Source: CAD feature listing. Evaluate the final solid. Frame: model axes, mm. Round coordinates to 2 decimals unless told otherwise and drop trailing zeros. Loops run counter-clockwise (first coordinate to the right, second up) from the corner with the lowest first, then second, coordinate; pieces in that order, holes last.
(1) Section A-A, the plane x = 55. Return the cut outline in (y, z).
(2) First-contact query: pin 1 Ø0.6 at (x, z) = (119, 13) entering from +Y. Flat tip, straight axial feed; report the tip coordinate or a pass-through.
(3) Section B-B, the plane z = 3.25. Return the cut outline in (x, y).
(4) Material intervals for probe 1 along X at (y, z) = (15.25, 2.25); probe 2 along Z at (x, y) = (36, 10.5); probe 3 along Z at (x, y) = (24.5, 0.5), sorted ascending.
```python
from build123d import *

# Parameters (mm, degrees)
SKETCH1_W           = 22
SKETCH1_H           = 18
BOSS_EXTRUDE1_DEPTH = 20
SKETCH2_W           = 12
SKETCH2_H           = 10
CUT_EXTRUDE1_DEPTH  = 13
SKETCH3_W           = 20
SKETCH3_H           = 5
BOSS_EXTRUDE2_DEPTH = 2
LPATTERN1_COUNT     = 6
LPATTERN1_PITCH     = 24
SKETCH4_W           = 20
SKETCH4_H           = 13
BOSS_EXTRUDE3_DEPTH = 2
SKETCH5_W           = 20
SKETCH5_H           = 18
BOSS_EXTRUDE4_DEPTH = 2
SKETCH6_W           = 132
SKETCH6_H           = 2
CUT_EXTRUDE2_DEPTH  = 2
SKETCH7_W           = 146
SKETCH7_H           = 20
BOSS_EXTRUDE5_DEPTH = 6


with BuildPart() as part:
    # Sketch1 → Boss-Extrude1 (new body)
    with BuildSketch(Plane.XY):
        with Locations((11, 9)):
            Rectangle(SKETCH1_W, SKETCH1_H)
    extrude(amount=BOSS_EXTRUDE1_DEPTH)

    # Sketch2 → Cut-Extrude1 (cut)
    with BuildSketch(Plane.XZ):
        with Locations((11, 10)):
            Rectangle(SKETCH2_W, SKETCH2_H)
    extrude(amount=-CUT_EXTRUDE1_DEPTH, mode=Mode.SUBTRACT)

    # Sketch3 → Boss-Extrude2 (add)
    with BuildSketch(Plane(origin=(22, 0, 0), x_dir=(0, 0, -1), z_dir=(1, 0, 0))):
        with Locations((-10, 2.5)):
            Rectangle(SKETCH3_W, SKETCH3_H)
    extrude(amount=BOSS_EXTRUDE2_DEPTH)


with BuildPart() as lpattern1_1:
    # LPattern1: pattern copy
    add(part.part.moved(Location(Vector(1, 0, 0) * (1 * LPATTERN1_PITCH))))


with BuildPart() as lpattern1_2:
    # LPattern1: pattern copy
    add(part.part.moved(Location(Vector(1, 0, 0) * (2 * LPATTERN1_PITCH))))


with BuildPart() as lpattern1_3:
    # LPattern1: pattern copy
    add(part.part.moved(Location(Vector(1, 0, 0) * (3 * LPATTERN1_PITCH))))


with BuildPart() as lpattern1_4:
    # LPattern1: pattern copy
    add(part.part.moved(Location(Vector(1, 0, 0) * (4 * LPATTERN1_PITCH))))


with BuildPart() as lpattern1_5:
    # LPattern1: pattern copy
    add(part.part.moved(Location(Vector(1, 0, 0) * (5 * LPATTERN1_PITCH))))

    # Sketch4 → Boss-Extrude3 (add)
    with BuildSketch(Plane(origin=(142, 0, 0), x_dir=(0, 0, -1), z_dir=(1, 0, 0))):
        with Locations((-10, 11.5)):
            Rectangle(SKETCH4_W, SKETCH4_H)
    extrude(amount=BOSS_EXTRUDE3_DEPTH)


with BuildPart() as part_1:
    add(part.part)

    # Sketch5 → Boss-Extrude4 (add)
    with BuildSketch(Plane.ZY):
        with Locations((10, 9)):
            Rectangle(SKETCH5_W, SKETCH5_H)
    extrude(amount=BOSS_EXTRUDE4_DEPTH)


with BuildPart() as lpattern1_1_1:
    add(lpattern1_1.part)

    # Combine1: union LPattern1_2, LPattern1_3, LPattern1_4, LPattern1_5, part
    add(lpattern1_2.part)
    add(lpattern1_3.part)
    add(lpattern1_4.part)
    add(lpattern1_5.part)
    add(part_1.part)

    # Sketch6 → Cut-Extrude2 (cut)
    with BuildSketch(Plane(origin=(0, 0, 0), x_dir=(-1, 0, 0), z_dir=(0, -1, 0))):
        with Locations((-71, -10)):
            Rectangle(SKETCH6_W, SKETCH6_H)
    extrude(amount=-CUT_EXTRUDE2_DEPTH, mode=Mode.SUBTRACT)

    # Sketch7 → Boss-Extrude5 (add)
    with BuildSketch(Plane(origin=(0, 0, 0), x_dir=(-1, 0, 0), z_dir=(0, -1, 0))):
        with Locations((-71, -10)):
            Rectangle(SKETCH7_W, SKETCH7_H)
    extrude(amount=BOSS_EXTRUDE5_DEPTH)


solid = lpattern1_1_1.part
```
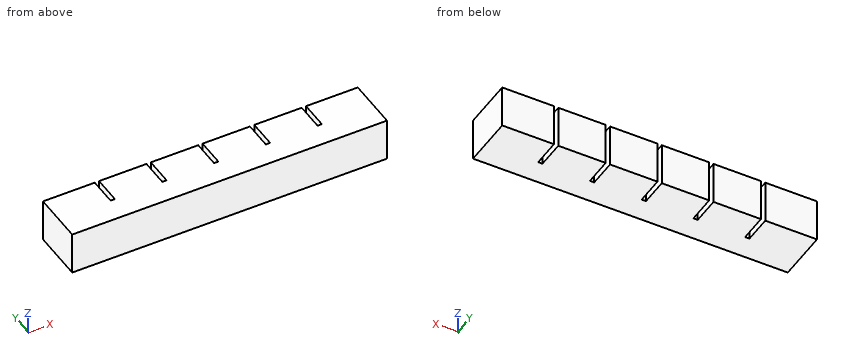
Output values:
1. outline: (-6, 0) - (18, 0) - (18, 20) - (-6, 20) - close; hole (0, 5) - (13, 5) - (13, 15) - (0, 15) - close
2. pin 1: stops at y = 5
3. outline: (-2, -6) - (144, -6) - (144, 18) - (120, 18) - (120, 5) - (118, 5) - (118, 18) - (96, 18) - (96, 5) - (94, 5) - (94, 18) - (72, 18) - (72, 5) - (70, 5) - (70, 18) - (48, 18) - (48, 5) - (46, 5) - (46, 18) - (24, 18) - (24, 5) - (22, 5) - (22, 18) - (-2, 18) - close
4. probe 1: x = -2 to 22, 24 to 46, 48 to 70, 72 to 94, 96 to 118, 120 to 144
4. probe 2: z = 0 to 5, 15 to 20
4. probe 3: z = 0 to 9, 11 to 20
